Can you work these out from the drawing? Everything is in mm from the part's minimum corner. A direction names the side the tool comes from. Coordinates: 2 decimals unless noted, no trailing zeros. Order: outer loops, then holes, each group sorted by start corner. A loop starts at its lowest first (then second) coordinate and runs counter-clockwise, first axis right, second up. Notation, with made-up numbers: (82.5, 75.5) - (117.5, 75.5) arc R16 cw to (117.5, 80.5) - close; hole circle Ø8 at (62.25, -7.5). An arc over 180 degrees is marked (long way). Use one line per item in the form item = value. Start each with the question number.
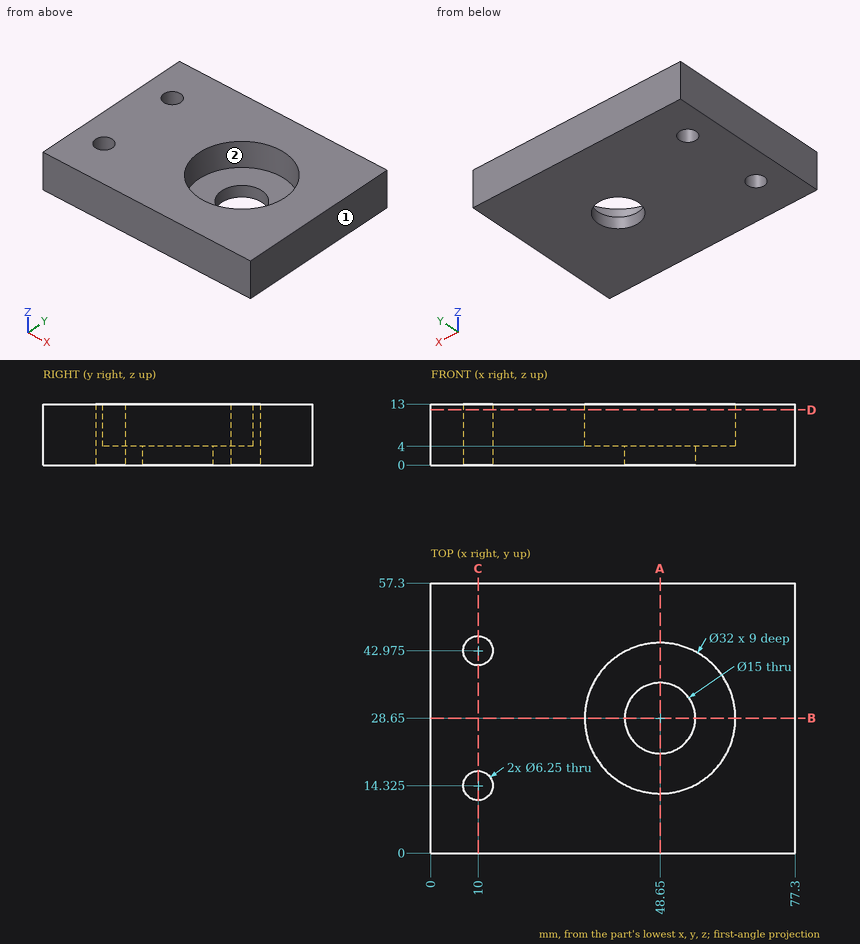
1) Which directions (+Z, -Z, +X, -X, +Y, -Y) give clear straight access to the entire face, cutting with the end or side of a thin tool? Please do the marked faces 1 and 2.
2) Suppose I cut it at A-A, the plane x = 48.65. List the corners of the cut face in (y, z) for me, then the cut area to 3 significant figures.
3) For pin 1 (9.5 mm diameter, centred on x = 50.5, y = 25, fed in from +Z), with a flat end and sliding along its axis, tell me the tip position at first contact or that it passes through.
4) Suppose I cut it at B-B, the plane y = 28.65. List the corners of the cut face in (x, z) for me.
5) Suppose I cut it at D-D, the plane z = 11.75. List the corners of the cut face in (x, y) for me (3 decimals).
6) Suppose I cut it at C-C, the plane x = 10. List the corners of the cut face in (y, z) for me.
7) I need wall thicknesses on probe 1 along Y at (x, z) = (10, 9); probe 2 along X at (y, z) = (17, 7.5); probe 3 along X at (y, z) = (29, 12). Which ranges of each line are inside material? Lowest first, please. Write a range as [from, to].
From the geometry:
q1.face_1 = +Z, -Z, +X, +Y, -Y
q1.face_2 = +Z
q2.outline = (0, 0) - (21.15, 0) - (21.15, 4) - (12.65, 4) - (12.65, 13) - (0, 13) - close; (36.15, 0) - (57.3, 0) - (57.3, 13) - (44.65, 13) - (44.65, 4) - (36.15, 4) - close
q2.area = 397 mm2
q3.pin_1 = 4
q4.outline = (0, 0) - (41.15, 0) - (41.15, 4) - (32.65, 4) - (32.65, 13) - (0, 13) - close; (56.15, 0) - (77.3, 0) - (77.3, 13) - (64.65, 13) - (64.65, 4) - (56.15, 4) - close
q5.outline = (0, 0) - (77.3, 0) - (77.3, 57.3) - (0, 57.3) - close; hole circle Ø6.25 at (10, 14.325); hole circle Ø6.25 at (10, 42.975); hole circle Ø32 at (48.65, 28.65)
q6.outline = (0, 0) - (11.2, 0) - (11.2, 13) - (0, 13) - close; (17.45, 0) - (39.85, 0) - (39.85, 13) - (17.45, 13) - close; (46.1, 0) - (57.3, 0) - (57.3, 13) - (46.1, 13) - close
q7.probe_1 = [0, 11.2], [17.45, 39.85], [46.1, 57.3]
q7.probe_2 = [0, 8.38], [11.62, 37.68], [59.62, 77.3]
q7.probe_3 = [0, 32.65], [64.65, 77.3]
